from build123d import *

# Parameters (mm, degrees)
SKETCH1_R          = 1.5875
EXTRUDE1_DEPTH     = 3.81
SKETCH2_R          = 3.81
EXTRUDE2_DEPTH     = 7.62
SKETCH3_R          = 11.43
EXTRUDE3_DEPTH     = 6.35
SKETCH4_R          = 12.065
EXTRUDE4_DEPTH     = 1.27
SKETCH5_R          = 7
EXTRUDE5_DEPTH     = 14.5
SKETCH6_R          = 7.5
EXTRUDE6_DEPTH     = 13.3
SKETCH7_R          = 7.239
EXTRUDE7_DEPTH     = 2.54
CHAMFER6_SIZE      = 0.762
SKETCH8_R          = 6.477
EXTRUDE8_DEPTH     = 3.81
SKETCH9_R          = 0.79375
CUT_EXTRUDE1_DEPTH = 2.54
CHAMFER1_SIZE      = 1.27
CHAMFER1_SIZE2     = 0.462242198
SKETCH10_R         = 7.518539915
EXTRUDE9_DEPTH     = 1.524
SKETCH11_R         = 6.35
EXTRUDE10_DEPTH    = 4.064
FILLET1_R          = 0.254
CHAMFER7_SIZE      = 0.762
EXTRUDE11_DEPTH    = 8.509
SKETCH13_W         = 13.97
SKETCH13_H         = 8.89
CUT_EXTRUDE2_DEPTH = 10.414
SKETCH14_W         = 2.763435098
SKETCH14_H         = 1.082967808
SKETCH14_W_2       = 3.024841121
EXTRUDE12_DEPTH    = 6.35
CHAMFER8_SIZE      = 0.762
FILLET2_R          = 2.54
FILLET3_R          = 0.635
EXTRUDE13_DEPTH    = 4.445


with BuildPart() as part:
    # Sketch1 → Extrude1 (new body)
    with BuildSketch(Plane(origin=(0, 0, 0), x_dir=(1, 0, 0), z_dir=(0, 1, 0))):
        with Locations(Location((0, 0, 0), (0, 0, 90))):
            Circle(SKETCH1_R)
    extrude(amount=EXTRUDE1_DEPTH)

    # Sketch2 → Extrude2 (add)
    with BuildSketch(Plane(origin=(0, 3.81, 0), x_dir=(1, 0, 0), z_dir=(0, 1, 0))):
        with Locations(Location((0, 0, 0), (0, 0, 90))):
            Circle(SKETCH2_R)
    extrude(amount=EXTRUDE2_DEPTH)

    # Sketch3 → Extrude3 (add)
    with BuildSketch(Plane(origin=(0, 11.43, 0), x_dir=(1, 0, 0), z_dir=(0, 1, 0))):
        with Locations(Location((0, 0, 0), (0, 0, 270))):
            Circle(SKETCH3_R)
    extrude(amount=EXTRUDE3_DEPTH)

    # Sketch4 → Extrude4 (add)
    with BuildSketch(Plane(origin=(0, 17.78, 0), x_dir=(1, 0, 0), z_dir=(0, 1, 0))):
        with Locations(Location((0, 0, 0), (0, 0, 270))):
            Circle(SKETCH4_R)
    extrude(amount=EXTRUDE4_DEPTH)

    # Sketch5 → Extrude5 (add)
    with BuildSketch(Plane(origin=(0, 19.05, 0), x_dir=(1, 0, 0), z_dir=(0, 1, 0))):
        with Locations(Location((0, 0, 0), (0, 0, 90))):
            Circle(SKETCH5_R)
    extrude(amount=EXTRUDE5_DEPTH)

    # Sketch6 → Extrude6 (add)
    with BuildSketch(Plane(origin=(0, 33.55, 0), x_dir=(1, 0, 0), z_dir=(0, 1, 0))):
        with Locations(Location((0, 0, 0), (0, 0, 270))):
            Circle(SKETCH6_R)
    extrude(amount=EXTRUDE6_DEPTH)

    # Sketch7 → Extrude7 (add)
    with BuildSketch(Plane(origin=(0, 46.85, 0), x_dir=(1, 0, 0), z_dir=(0, 1, 0))):
        with Locations(Location((0, 0, 0), (0, 0, 270))):
            Circle(SKETCH7_R)
    extrude(amount=EXTRUDE7_DEPTH)

    # Chamfer6
    chamfer6_edges = [part.edges().sort_by_distance(p)[0] for p in [
        (0, 49.39, -7.239),
    ]]
    chamfer(chamfer6_edges, length=CHAMFER6_SIZE)

    # Sketch8 → Extrude8 (add)
    with BuildSketch(Plane(origin=(0, 49.39, 0), x_dir=(1, 0, 0), z_dir=(0, 1, 0))):
        with Locations(Location((0, 0, 0), (0, 0, 90))):
            Circle(SKETCH8_R)
    extrude(amount=EXTRUDE8_DEPTH)

    # Sketch9 → Cut-Extrude1 (cut)
    with BuildSketch(Plane.XZ):
        with Locations(Location((0, 0, 0), (0, 0, 270))):
            Circle(SKETCH9_R)
    extrude(amount=-CUT_EXTRUDE1_DEPTH, mode=Mode.SUBTRACT)

    # Chamfer1
    chamfer1_edges = [part.edges().sort_by_distance(p)[0] for p in [
        (0, 0, 0.79375),
    ]]
    chamfer1_side = [part.faces().sort_by_distance(p)[0] for p in [
        (0, 1.27, 0.79375),
    ]]
    chamfer(chamfer1_edges, length=CHAMFER1_SIZE, length2=CHAMFER1_SIZE2, reference=chamfer1_side[0])

    # Sketch10 → Extrude9 (add)
    with BuildSketch(Plane(origin=(0, 53.2, 0), x_dir=(1, 0, 0), z_dir=(0, 1, 0))):
        with Locations(Location((0, 0, 0), (0, 0, 90))):
            Circle(SKETCH10_R)
    extrude(amount=EXTRUDE9_DEPTH)

    # Sketch11 → Extrude10 (add)
    with BuildSketch(Plane(origin=(0, 54.724, 0), x_dir=(1, 0, 0), z_dir=(0, 1, 0))):
        with Locations(Location((0, 0, 0), (0, 0, 270))):
            Circle(SKETCH11_R)
    extrude(amount=EXTRUDE10_DEPTH)

    # Fillet1
    fillet1_edges = [part.edges().sort_by_distance(p)[0] for p in [
        (0, 19.05, 7),
    ]]
    fillet(fillet1_edges, radius=FILLET1_R)

    # Chamfer7
    chamfer7_edges = [part.edges().sort_by_distance(p)[0] for p in [
        (0, 11.43, -11.43),
    ]]
    chamfer(chamfer7_edges, length=CHAMFER7_SIZE)

    # Sketch12 → Extrude11 (add, symmetric)
    with BuildSketch(Plane(origin=(0, 0, 0), x_dir=(0, 0, -1), z_dir=(1, 0, 0))):
        Polygon((-4.0005, 33.55), (-4.0005, 46.993498834), (4.0005, 46.993498834), (4.0005, 39.645358569), (14.608417816, 50.253276385), (23.049858569, 41.811835631), (14.788022938, 33.55), (10.4775, 37.860522938), (10.4775, 33.55), align=None)
    extrude(amount=EXTRUDE11_DEPTH, both=True)

    # Sketch13 → Cut-Extrude2 (cut)
    with BuildSketch(Plane(origin=(0, 32.4308471, -32.4308471), x_dir=(1, 0, 0), z_dir=(0, 0.7071067811865482, -0.7071067811865468))):
        with Locations((0, -19.235721209)):
            Rectangle(SKETCH13_W, SKETCH13_H)
    extrude(amount=-CUT_EXTRUDE2_DEPTH, mode=Mode.SUBTRACT)

    # Sketch14 → Extrude12 (add)
    with BuildSketch(Plane(origin=(0, 25.067037081, -25.067037081), x_dir=(1, 0, 0), z_dir=(0, 0.7071067811865475, -0.7071067811865477))):
        with Locations((-3.379408051, -24.201118939)):
            Rectangle(SKETCH14_W, SKETCH14_H)
        with Locations((2.091446569, -24.201118939)):
            Rectangle(SKETCH14_W_2, SKETCH14_H)
    extrude(amount=EXTRUDE12_DEPTH)

    # Chamfer8
    chamfer8_edges = [part.edges().sort_by_distance(p)[0] for p in [
        (-1.997690502, 46.294508604, -12.81982168),
        (-4.7611256, 46.294508604, -12.81982168),
        (3.60386713, 46.294508604, -12.81982168),
        (0.579026009, 46.294508604, -12.81982168),
    ]]
    chamfer(chamfer8_edges, length=CHAMFER8_SIZE)

    # Fillet2
    fillet2_edges = [part.edges().sort_by_distance(p)[0] for p in [
        (-8.509, 37.680917816, -18.918940754),
        (8.509, 37.680917816, -18.918940754),
        (6.985, 39.207561356, -18.290322825),
        (-6.985, 39.207561356, -18.290322825),
        (-6.985, 45.493740641, -12.004143541),
        (6.985, 45.493740641, -12.004143541),
    ]]
    fillet(fillet2_edges, radius=FILLET2_R)

    # Fillet3
    fillet3_edges = [part.edges().sort_by_distance(p)[0] for p in [
        (-8.509, 44.949317477, -9.304458908),
        (8.509, 44.949317477, -9.304458908),
    ]]
    fillet(fillet3_edges, radius=FILLET3_R)

    # Sketch15 → Extrude13 (add, symmetric)
    with BuildSketch(Plane(origin=(0, 0, 0), x_dir=(0, 0, -1), z_dir=(1, 0, 0))):
        Polygon((5.360156527, 46.85), (12.103167043, 46.85), (5.360156527, 41.005015096), align=None)
        Polygon((10.4775, 33.55), (14.788022938, 33.55), (10.4775, 37.860522938), align=None)
    extrude(amount=EXTRUDE13_DEPTH, both=True)


solid = part.part
The model under review builds one solid part; all positions refer to its coordinate system, in mm. A direction names the side the tool comes from. Round coordinates to 2 decimals unless told otherwise and drop trailing zeros. Use one line per item in the form item = value.
Q1. Clearance check with flat-ended pins moving along their axes: P1, Ø5, axis at x = -4.5, z = 7, coming from the -Y side; P2, Ø13, axis at y = 44, z = -14.5, coming from the -X side; P3, Ø5, axis at x = 3.5, y = 36, coming from the +Z side. State where each tip first meets the part, or that it passes through.
Response values:
P1 = 11.43
P2 = -8.51
P3 = 7.43
Q2. To check wall thickness, follow line 1 (X direction, y = 1.7, z = 0); line 2 (Y direction, x = -1, z = -9.5); line 3 (Y direction, x = 0.5, z = -9). State the ranges of each line that lie inside material, in increasing order.
Response values:
line_1 = -1.59 to -0.79, 0.79 to 1.59
line_2 = 11.43 to 19.05, 33.55 to 40.63, 42.99 to 46.85
line_3 = 11.43 to 19.05, 33.55 to 41.13, 42.49 to 46.85
Q3. Tool access review of faces 1 (the flat face through (-4, 17.78, 11)), 2 (the flat face through (8.509, 40, -6)), 3 (the flat face through (4.445, 35, -12)): name each direction out of +Z, -Z, +X, -X, +Y, -Y from which nothing blocks a thin tool from reaching the whole face with its end or side.
Response values:
face_1 = -Y
face_2 = +Z, -Z, +X, +Y
face_3 = +X
Q4. Mouldability with a two-part tool opening along Y and no side actions: class faces 4 (the flat face through (0, 2.54, 0)), 5 (the cylindrical face through (8.318, 44.674, -9.285)), 6 (the flat face through (-8, 19.05, 0)) as pulls with the +Y half, pulls with the -Y half, needs draft (parallel to the pull), parting line crosses it, or undercut.
Response values:
face_4 = pulls with the -Y half
face_5 = pulls with the +Y half
face_6 = undercut
